Could you check a few things on this model? Use its own coordinates, in mm. Face numbers are marked on the shaded views. Round coordinates to 2 decimals unless told otherwise and drop trailing zeros. Loops run counter-clockwise (first coordinate to the right, second up) from the corner with the lowest first, then second, coordinate; pieces in that order, holes last. Notation, with made-up numbers: (9.5, 8) -> (37.5, 8) arc R24 ccw to (37.5, 22) -> close; hole circle Ø6 at (82.5, -39.75). An arc over 180 degrees is marked (long way). Put each result on its own line as item: value. Start each with the question number.
1. If we mould it in two halves opening along Y, with no side actions, what happens to the marked faces 1 and 2? For each: pulls with the +Y half, pulls with the -Y half, needs draft (parallel to the pull), parting line crosses it, or undercut.
2. Imagine slicing it at B-B, the plane y = 0. Please give me the cut outline in (x, z), and give its area (3 significant figures).
3. I need wall thicknesses on line 1 (Y direction, x = 0, z = 1.05); line 2 (X direction, y = 2.5, z = 1.2); line 3 (Z direction, x = 6, y = 5.5). Which ranges of each line are inside material? Lowest first, please. Write a range as [from, to].
4. Imagine slicing it at C-C, the plane y = 12.5. Please give me the cut outline in (x, z) (3 decimals), and give its area (3 significant figures).
5. Imagine slicing it at A-A, the plane y = 25.5. Please give me the cut outline in (x, z) (3 decimals).
6. I'm going to push flat-ended pins straight in: P1, Ø1.4, axis at y = 19.5, z = 2.5, coming from the -X side; P2, Ø1.3, axis at y = 0.5, z = 0.5, coming from the +X side; P3, Ø1, axis at x = 19.5, z = 2, coming from the -Y side; P4, Ø0.6, axis at x = 16, z = 2, coming from the +Y side. Where does each tip first touch, or does it pass through?
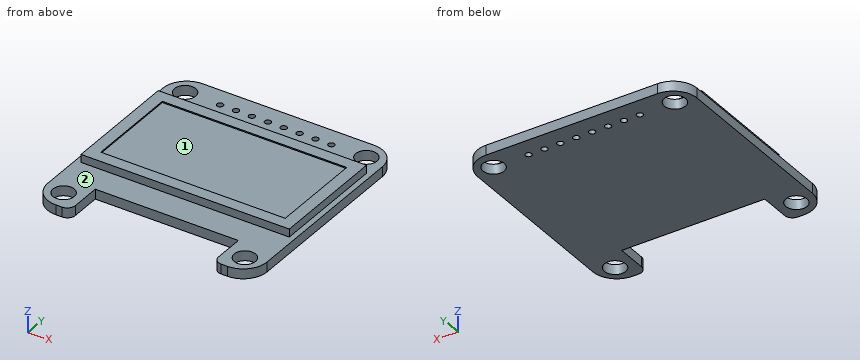
```python
from build123d import *

# Parameters (mm, degrees)
SKETCH2_W                = 35.052
SKETCH2_H                = 35.56
BOSS_EXTRUDE1_DEPTH      = 1.5748
CUT_EXTRUDE4_START       = 1.5748
SKETCH2_8_W              = 22.86
SKETCH2_8_H              = 6.096
CUT_EXTRUDE4_DEPTH       = 1.5748
M3_CLEARANCE_HOLE1_D     = 3.4
F_1_0_1_DIAMETER_HOLE1_D = 1
FILLET2_R                = 3.81
FILLET3_R                = 1.27
SKETCH10_W               = 33.274
SKETCH10_H               = 18.731056846
BOSS_EXTRUDE2_DEPTH      = 1.27
SKETCH11_W               = 29.464
SKETCH11_H               = 14.921056846
CUT_EXTRUDE5_DEPTH       = 0.1905


with BuildPart() as part:
    # Sketch2 → Boss-Extrude1 (new body)
    with BuildSketch(Plane.XY):
        with Locations((14.478, 14.732)):
            Rectangle(SKETCH2_W, SKETCH2_H)
    extrude(amount=BOSS_EXTRUDE1_DEPTH)

    # Sketch2<8> → Cut-Extrude4 (cut)
    with BuildSketch(Plane.XY.offset(CUT_EXTRUDE4_START)):
        with Locations((14.478, 0)):
            Rectangle(SKETCH2_8_W, SKETCH2_8_H)
    extrude(amount=-CUT_EXTRUDE4_DEPTH, mode=Mode.SUBTRACT)

    # M3 Clearance Hole1 (through all)
    with Locations(Plane.XY.offset(1.5748)):
        with Locations((0, 29.464), (0, 0), (28.956, 0), (28.956, 29.464)):
            Hole(M3_CLEARANCE_HOLE1_D / 2)

    # Ø1.0 (1) Diameter Hole1 (through all)
    with Locations(Plane.XY.offset(1.5748)):
        with Locations((5.588, 29.464), (8.128, 29.464), (10.668, 29.464), (13.208, 29.464), (15.748, 29.464), (18.288, 29.464), (20.828, 29.464), (23.368, 29.464)):
            Hole(F_1_0_1_DIAMETER_HOLE1_D / 2)

    # Fillet2
    fillet2_edges = [part.edges().sort_by_distance(p)[0] for p in [
        (-3.048, 32.512, 0.7874),
        (-3.048, -3.048, 0.7874),
        (32.004, -3.048, 0.7874),
        (32.004, 32.512, 0.7874),
    ]]
    fillet(fillet2_edges, radius=FILLET2_R)

    # Fillet3
    fillet3_edges = [part.edges().sort_by_distance(p)[0] for p in [
        (25.908, -3.048, 0.7874),
        (3.048, -3.048, 0.7874),
    ]]
    fillet(fillet3_edges, radius=FILLET3_R)

    # Sketch10 → Boss-Extrude2 (add)
    with BuildSketch(Plane.XY.offset(1.5748)):
        with Locations((14.478, 16.858528423)):
            Rectangle(SKETCH10_W, SKETCH10_H)
    extrude(amount=BOSS_EXTRUDE2_DEPTH)

    # Sketch11 → Cut-Extrude5 (cut)
    with BuildSketch(Plane.XY.offset(2.8448)):
        with Locations((14.478, 16.858528423)):
            Rectangle(SKETCH11_W, SKETCH11_H)
    extrude(amount=-CUT_EXTRUDE5_DEPTH, mode=Mode.SUBTRACT)


solid = part.part
```
Entries:
1. face 1: undercut
1. face 2: needs draft
2. outline: (-2.97, 0) -> (-1.7, 0) -> (-1.7, 1.57) -> (-2.97, 1.57) -> close; (1.7, 0) -> (3.05, 0) -> (3.05, 1.57) -> (1.7, 1.57) -> close; (25.91, 0) -> (27.26, 0) -> (27.26, 1.57) -> (25.91, 1.57) -> close; (30.66, 0) -> (31.93, 0) -> (31.93, 1.57) -> (30.66, 1.57) -> close
2. area: 8.25 mm^2
3. line 1: [-2.97, -1.7], [1.7, 27.76], [31.16, 32.44]
3. line 2: [-3.05, 3.05], [25.91, 32]
3. line 3: [0, 1.57]
4. outline: (-3.048, 0) -> (32.004, 0) -> (32.004, 1.575) -> (31.115, 1.575) -> (31.115, 2.845) -> (29.21, 2.845) -> (29.21, 2.654) -> (-0.254, 2.654) -> (-0.254, 2.845) -> (-2.159, 2.845) -> (-2.159, 1.575) -> (-3.048, 1.575) -> close
4. area: 91.8 mm^2
5. outline: (-3.048, 0) -> (32.004, 0) -> (32.004, 1.575) -> (31.115, 1.575) -> (31.115, 2.845) -> (-2.159, 2.845) -> (-2.159, 1.575) -> (-3.048, 1.575) -> close
6. P1: x = -2.16
6. P2: x = 32
6. P3: y = 3.05
6. P4: y = 26.22
